```python
from build123d import *

# Parameters (mm, degrees)
EXTRUDE_1_DEPTH             = 120
HOLE_WIZARD_8_5_8_5_1_D     = 8.5
PATTERN_LINEAR_1_COUNT      = 2
PATTERN_LINEAR_1_PITCH      = 190
PATTERN_LINEAR_1_COUNT_DIR2 = 2
PATTERN_LINEAR_1_PITCH_DIR2 = 80
CUT_EXTRUDE_2_REACH         = 244.332
SKETCH_3_R                  = 40


with BuildPart() as part:
    # 草图1 → 拉伸1 (new body)
    with BuildSketch(Plane.XY):
        Polygon((0, 0), (210, 0), (210, 10), (190, 10), (190, 15), (20, 15), (20, 10), (0, 10), align=None)
    extrude(amount=EXTRUDE_1_DEPTH)

    # Ø8.5 (8.5) 直径孔1 (through all)
    with Locations(Plane(origin=(10, 0, 20), x_dir=(0, 0, -1), z_dir=(0, -1, 0))):
        with Locations((0, 0)):
            hole_wizard_8_5_8_5_1 = Hole(HOLE_WIZARD_8_5_8_5_1_D / 2)

    # 阵列(线性)1: Hole Wizard 8.5 _8.5_ _1 2 × 2
    with Locations(*[(i * PATTERN_LINEAR_1_PITCH, 0, j * PATTERN_LINEAR_1_PITCH_DIR2) for i in range(PATTERN_LINEAR_1_COUNT) for j in range(PATTERN_LINEAR_1_COUNT_DIR2) if (i, j) != (0, 0)]):
        add(hole_wizard_8_5_8_5_1, mode=Mode.SUBTRACT)

    # 草图3 → 拉伸2 (cut, up to next)
    with BuildSketch(Plane.XZ, mode=Mode.PRIVATE) as cut_extrude_2_sk1:
        with Locations(Location((105, 60, 0), (0, 0, 270))):
            Circle(SKETCH_3_R)
    cut_extrude_2_tool1 = extrude(cut_extrude_2_sk1.sketch, amount=-CUT_EXTRUDE_2_REACH, mode=Mode.PRIVATE) & part.part
    # 草图3 → 拉伸2 (cut, up to next)
    with BuildSketch(Plane.XZ, mode=Mode.PRIVATE) as cut_extrude_2_sk2:
        with BuildLine():
            Line((45.75, 96), (45.75, 76))
            ThreePointArc((45.75, 76), (50, 71.75), (54.25, 76))
            Line((54.25, 76), (54.25, 96))
            ThreePointArc((54.25, 96), (50, 100.25), (45.75, 96))
        make_face()
    cut_extrude_2_tool2 = extrude(cut_extrude_2_sk2.sketch, amount=-CUT_EXTRUDE_2_REACH, mode=Mode.PRIVATE) & part.part
    # 草图3 → 拉伸2 (cut, up to next)
    with BuildSketch(Plane.XZ, mode=Mode.PRIVATE) as cut_extrude_2_sk3:
        with BuildLine():
            Line((155.75, 96), (155.75, 76))
            ThreePointArc((155.75, 76), (160, 71.75), (164.25, 76))
            Line((164.25, 76), (164.25, 96))
            ThreePointArc((164.25, 96), (160, 100.25), (155.75, 96))
        make_face()
    cut_extrude_2_tool3 = extrude(cut_extrude_2_sk3.sketch, amount=-CUT_EXTRUDE_2_REACH, mode=Mode.PRIVATE) & part.part
    # 草图3 → 拉伸2 (cut, up to next)
    with BuildSketch(Plane.XZ, mode=Mode.PRIVATE) as cut_extrude_2_sk4:
        with BuildLine():
            Line((45.75, 60), (45.75, 40))
            ThreePointArc((45.75, 40), (50, 35.75), (54.25, 40))
            Line((54.25, 40), (54.25, 60))
            ThreePointArc((54.25, 60), (50, 64.25), (45.75, 60))
        make_face()
    cut_extrude_2_tool4 = extrude(cut_extrude_2_sk4.sketch, amount=-CUT_EXTRUDE_2_REACH, mode=Mode.PRIVATE) & part.part
    # 草图3 → 拉伸2 (cut, up to next)
    with BuildSketch(Plane.XZ, mode=Mode.PRIVATE) as cut_extrude_2_sk5:
        with BuildLine():
            Line((155.75, 60), (155.75, 40))
            ThreePointArc((155.75, 40), (160, 35.75), (164.25, 40))
            Line((164.25, 40), (164.25, 60))
            ThreePointArc((164.25, 60), (160, 64.25), (155.75, 60))
        make_face()
    cut_extrude_2_tool5 = extrude(cut_extrude_2_sk5.sketch, amount=-CUT_EXTRUDE_2_REACH, mode=Mode.PRIVATE) & part.part
    add(cut_extrude_2_tool1.solids().sort_by_distance((105, 0, 60))[0], mode=Mode.SUBTRACT)
    add(cut_extrude_2_tool2.solids().sort_by_distance((50, 0, 86))[0], mode=Mode.SUBTRACT)
    add(cut_extrude_2_tool3.solids().sort_by_distance((160, 0, 86))[0], mode=Mode.SUBTRACT)
    add(cut_extrude_2_tool4.solids().sort_by_distance((50, 0, 50))[0], mode=Mode.SUBTRACT)
    add(cut_extrude_2_tool5.solids().sort_by_distance((160, 0, 50))[0], mode=Mode.SUBTRACT)


solid = part.part
```
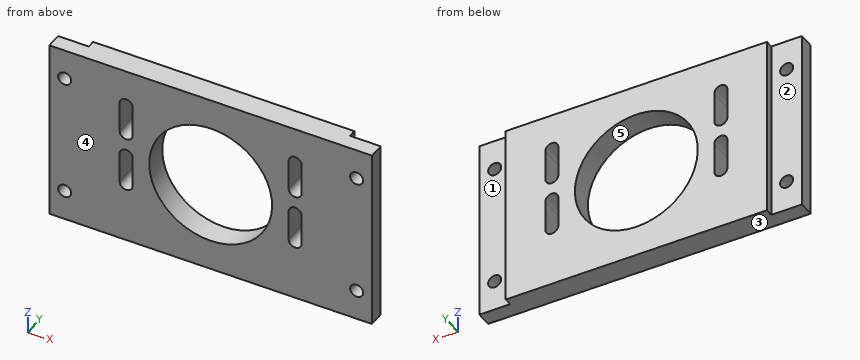
Here's how the part is built. I have some questions about the finished solid (model axes, mm). Face numbers are marked on the shaded views. A direction names the side the tool comes from. Coordinates: 2 decimals unless noted, no trailing zeros. Order: outer loops, then holes, each group sorted by start corner. A loop starts at its lowest first (then second) coordinate and runs counter-clockwise, first axis right, second up. Notation, with made-up numbers: (32.25, -34.75) - (45.25, -34.75) arc R19 ccw to (45.25, -14.75) - close; hole circle Ø2 at (12.25, 17.5). An arc over 180 degrees is marked (long way). One line per question, with ' | ' between items. Start each with the question number.
1. I'm going to push flat-ended pins straight in: pin 1 Ø4 at (y, z) = (12.5, 68.5) entering from +X; pin 2 Ø10 at (x, z) = (10, 20) entering from +Y. Where does each tip first touch, or does it pass through?
2. If we mould it in two halves opening along X, with no side actions, what happens to the marked faces 4 and 5? For each: released by +X, released by -X, zero draft, split by the parting line, or undercut.
3. If we section it at B-B (x = 105): Write out the boundary of the cut face in (y, z), and give its area (3 significant figures).
4. Which directions (+Z, -Z, +X, -X, +Y, -Y) give clear straight access to the entire face, cutting with the end or side of a thin tool? Please do the marked faces 1, 2 and 3.
5. If we section it at C-C (y = 7): Give the number of separate pieces and of enclosed holes in the cut face, and give its area (3 significant figures).
6. Please list where these lines run through material, in increasing order: line 1 along X through (y, z) = (9, 60); line 2 along X through (y, z) = (4, 82); line 3 along Z through (x, y) = (158.5, 11.5). Write a range as [from, to].
7. If we section it at A-A (x = 200): Write out the boundary of the cut face in (y, z), and give its area (3 significant figures).
8. If we section it at D-D (z = 80.5): Write out the boundary of the cut face in (x, y).
Model answer:
1) pin 1: stops at x = 190 | pin 2: stops at y = 10
2) face 4: zero draft | face 5: undercut
3) outline: (0, 0) - (15, 0) - (15, 20) - (0, 20) - close; (0, 100) - (15, 100) - (15, 120) - (0, 120) - close | area: 600 mm²
4) face 1: +Z, -Z, +X, +Y | face 2: +Z, -Z, -X, +Y | face 3: -Z, +X, -X, +Y, -Y
5) separate pieces: 1 | enclosed holes: 9 | area: 19,000 mm²
6) line 1: x = [0, 45.75], [54.25, 65], [145, 155.75], [164.25, 210] | line 2: x = [0, 45.75], [54.25, 71.59], [138.41, 155.75], [164.25, 210] | line 3: z = [0, 36.02], [63.98, 72.02], [99.98, 120]
7) outline: (0, 0) - (10, 0) - (10, 15.75) - (0, 15.75) - close; (0, 24.25) - (10, 24.25) - (10, 95.75) - (0, 95.75) - close; (0, 104.25) - (10, 104.25) - (10, 120) - (0, 120) - close | area: 1,030 mm²
8) outline: (0, 0) - (45.75, 0) - (45.75, 15) - (20, 15) - (20, 10) - (0, 10) - close; (54.25, 0) - (70.65, 0) - (70.65, 15) - (54.25, 15) - close; (139.35, 0) - (155.75, 0) - (155.75, 15) - (139.35, 15) - close; (164.25, 0) - (210, 0) - (210, 10) - (190, 10) - (190, 15) - (164.25, 15) - close
